```python
from build123d import *

# Parameters (mm, degrees)
BOSS_EXTRUDE1_DEPTH = 29
BOSS_EXTRUDE3_START = -3
BOSS_EXTRUDE3_DEPTH = 3
BOSS_EXTRUDE4_DEPTH = 29
SKETCH6_W           = 15.595785808
SKETCH6_H           = 9.872798586
CUT_EXTRUDE1_DEPTH  = 2
BOSS_EXTRUDE5_DEPTH = 5


with BuildPart() as part:
    # Sketch2 → Boss-Extrude1 (new body)
    with BuildSketch(Plane(origin=(0, 0, 0), x_dir=(1, 0, 0), z_dir=(0, 1, 0))):
        with BuildLine():
            Line((-6, 6.020797289), (-6, 5))
            Line((-6, 5), (-5.921359641, 5))
            ThreePointArc((-5.921359641, 5), (0, 7.75), (5.921359641, 5))
            Line((5.921359641, 5), (6, 5))
            Line((6, 5), (6, 6.020797289))
            ThreePointArc((6, 6.020797289), (0, 8.5), (-6, 6.020797289))
        make_face()
    extrude(amount=BOSS_EXTRUDE1_DEPTH)

    # Sketch4 → Boss-Extrude3 (add)
    with BuildSketch(Plane(origin=(0, 21.1, 0), x_dir=(1, 0, 0), z_dir=(0, 1, 0)).offset(BOSS_EXTRUDE3_START)):
        with BuildLine():
            Line((6, 6.020797289), (6.006787511, 7.03427351))
            ThreePointArc((6.006787511, 7.03427351), (0.004460918, 9.249998925), (-6, 7.040063921))
            Line((-6, 7.040063921), (-6, 6.020797289))
            ThreePointArc((-6, 6.020797289), (0, 8.5), (6, 6.020797289))
        make_face()
    extrude(amount=BOSS_EXTRUDE3_DEPTH)

    # Sketch5 → Boss-Extrude4 (add)
    with BuildSketch(Plane.XZ):
        with BuildLine():
            Line((-5.921359641, -5), (5.921359641, -5))
            ThreePointArc((5.921359641, -5), (0, -7.75), (-5.921359641, -5))
        make_face()
    extrude(amount=-BOSS_EXTRUDE4_DEPTH)

    # Sketch6 → Cut-Extrude1 (cut)
    with BuildSketch(Plane.XZ):
        with Locations((-0.763992961, -6.245386966)):
            Rectangle(SKETCH6_W, SKETCH6_H)
    extrude(amount=-CUT_EXTRUDE1_DEPTH, mode=Mode.SUBTRACT)

    # Sketch7 → Boss-Extrude5 (add)
    with BuildSketch(Plane(origin=(0, 29, 0), x_dir=(1, 0, 0), z_dir=(0, 1, 0))):
        with BuildLine():
            Line((-6, 5), (6, 5))
            Line((6, 5), (6, 6.020797289))
            ThreePointArc((6, 6.020797289), (0, 8.5), (-6, 6.020797289))
            Line((-6, 6.020797289), (-6, 5))
        make_face()
    extrude(amount=BOSS_EXTRUDE5_DEPTH)


solid = part.part
```
Check sheet for the modelled part. Datum: model origin and axes. Units: mm. A direction names the side the tool comes from. Round coordinates to 2 decimals unless told otherwise and drop trailing zeros. Order: outer loops, then holes, each group sorted by start corner. A loop starts at its lowest first (then second) coordinate and runs counter-clockwise, first axis right, second up.
1) Section check A-A (x = 3.25). Record the boundary of the cut face in (y, z), and give its area (3 significant figures).
2) Section check D-D (x = 5). Record the boundary of the cut face in (y, z), and give its area (3 significant figures).
3) Scan lines: line 1 (X direction, y = 20, z = -5.2); line 2 (Z direction, x = 0.25, y = 4); line 3 (Z direction, x = -4.75, y = 29.5). Record each from-to range of solid material in increasing order.
4) Section check B-B (z = -6.6). Record the boundary of the cut face in (x, y).
5) Tool access check on faces 1 (the cylindrical face through (0.1, 9.9, -8.5)), 2 (the cylindrical face through (0.1, 27.5, -8.5)), 3 (the cylindrical face through (0.1, 19.58, -9.25)). Record the directions out of +Z, -Z, +X, -X, +Y, -Y that give a thin tool (end or side, any length) a straight path to the whole face; none if there is none.
6) Go/stop test with a flat-tipped pin: pin 1 Ø1 at (x, z) = (4.5, -7.5) entering from -Y. Record where the tip stops, or that it passes through.
7) Section check C-C (y = 18.5). Record the boundary of the cut face in (x, z), and give its area (3 significant figures).
Result:
1. outline: (2, -7.85) - (18.1, -7.85) - (18.1, -8.66) - (21.1, -8.66) - (21.1, -7.85) - (34, -7.85) - (34, -5) - (2, -5) - close
1. area: 93.8 mm2
2. outline: (2, -6.87) - (18.1, -6.87) - (18.1, -7.78) - (21.1, -7.78) - (21.1, -6.87) - (34, -6.87) - (34, -5) - (2, -5) - close
2. area: 62.7 mm2
3. line 1: x = -6 to 6
3. line 2: z = -8.5 to -5
3. line 3: z = -7.05 to -5
4. outline: (-6, 18.1) - (-5.36, 18.1) - (-5.36, 2) - (5.36, 2) - (5.36, 18.1) - (6, 18.1) - (6, 21.1) - (5.36, 21.1) - (5.36, 34) - (-5.36, 34) - (-5.36, 21.1) - (-6, 21.1) - close
5. face 1: -Z, -Y
5. face 2: -Z, +Y
5. face 3: -Z, +Y, -Y
6. pin 1: stops at y = 2
7. outline: (-6, -7.04) arc R9.25 ccw to (6.01, -7.03) - (6, -6.02) - (6, -5) - (-6, -5) - close
7. area: 42.6 mm2
